```python
from build123d import *

# Parameters (mm, degrees)
BOSS_EXTRUDE1_DEPTH = 100
BOSS_EXTRUDE2_DEPTH = 10


with BuildPart() as part:
    # Sketch1 → Boss-Extrude1 (new, symmetric)
    with BuildSketch(Plane.XY):
        Polygon((0, 0), (500, 0), (750, -310.66017178), align=None)
    extrude(amount=BOSS_EXTRUDE1_DEPTH, both=True)

    # Sketch2 → Boss-Extrude2 (add, symmetric)
    with BuildSketch(Plane.XY):
        Polygon((686.273799006, -284.263915049), (686.273799006, -231.471401589), (750, -291.408761965), (750, -310.66017178), align=None)
    extrude(amount=BOSS_EXTRUDE2_DEPTH, both=True)


solid = part.part
```
Work out the finished part from the listing and answer in its coordinate system (mm). A direction names the side the tool comes from. Coordinates: 2 decimals unless noted, no trailing zeros. Write each loop counter-clockwise with the first axis right and the second up, starting at its lowest first coordinate (ties: lowest second). Pieces come first, ordered by that corner, then holes.
Q1. Which of the six approach directions +Z, -Z, +X, -X, +Y, -Y give full straight-line access (tool end or side, diameter ignored) to faces 1 (the face through (728, -277, 10)), 2 (the face through (380, -119, -100))?
Q2. A cutting plane is placed at D-D, the plane y = -40. Give the vertices of the cut face in (x, z), then the cut area to 3 significant figures.
Q3. A cutting plane is placed at B-B, the plane z = -76. Give the vertices of the cut face in (x, y).
Q4. Each of these flat-tipped pins is pushed along its axis until it touches: pin 1 Ø2 at (y, z) = (-148.5, -73.5) entering from -X; pin 2 Ø6 at (x, z) = (442.5, -40) entering from -Y; pin 3 Ø12 at (y, z) = (-45.5, 35) entering from +X. Where does it stop, or does it pass through?
Q5. Find the intervals of material crossed by line 1 (X direction, y = -250.5, z = 80.5); line 2 (X direction, y = -74.5, z = -9); line 3 (Y direction, x = 272, z = 66), in increasing order.
Q6. A cutting plane is placed at A-A, the plane y = -249. Give the vertices of the cut face in (x, z), then the cut area to 3 significant figures.
Q7. A cutting plane is placed at C-C, the plane x = 704.5. Give the vertices of the cut face in (y, z), then the cut area to 3 significant figures.
Q8. Determine the mould class of faces 3 (the face through (728, -277, -10)), 4 (the face through (623.25, -153.155, 1.4)) for opening direction Y: released by +Y, released by -Y, zero draft, split by the parting line, or undercut.
Findings below:
1. face 1: +Z, +X, +Y
1. face 2: -Z, +X, -X, +Y, -Y
2. outline: (96.57, -100) - (532.19, -100) - (532.19, 100) - (96.57, 100) - close
2. area: 87,100 mm2
3. outline: (0, 0) - (750, -310.66) - (500, 0) - close
4. pin 1: stops at x = 356.1
4. pin 2: stops at y = -184.53
4. pin 3: stops at x = 541.44
5. line 1: x = 604.76 to 701.59
5. line 2: x = 179.86 to 559.95
5. line 3: y = -112.67 to 0
6. outline: (601.14, -100) - (700.38, -100) - (700.38, -10) - (704.91, -10) - (704.91, 10) - (700.38, 10) - (700.38, 100) - (601.14, 100) - close
6. area: 19,900 mm2
7. outline: (-291.81, -100) - (-254.12, -100) - (-254.12, -10) - (-248.61, -10) - (-248.61, 10) - (-254.12, 10) - (-254.12, 100) - (-291.81, 100) - close
7. area: 7,650 mm2
8. face 3: zero draft
8. face 4: released by +Y
